Part print with two shaded views. Sizes in mm from the minimum x, y, z corner. Give positions to 0.01 mm unless a question says otherwise; leave off trailing zeros. Write each loop counter-clockwise with the first axis right and the second up, starting at its lowest first coordinate (ties: lowest second). Pieces come first, ordered by that corner, then holes.
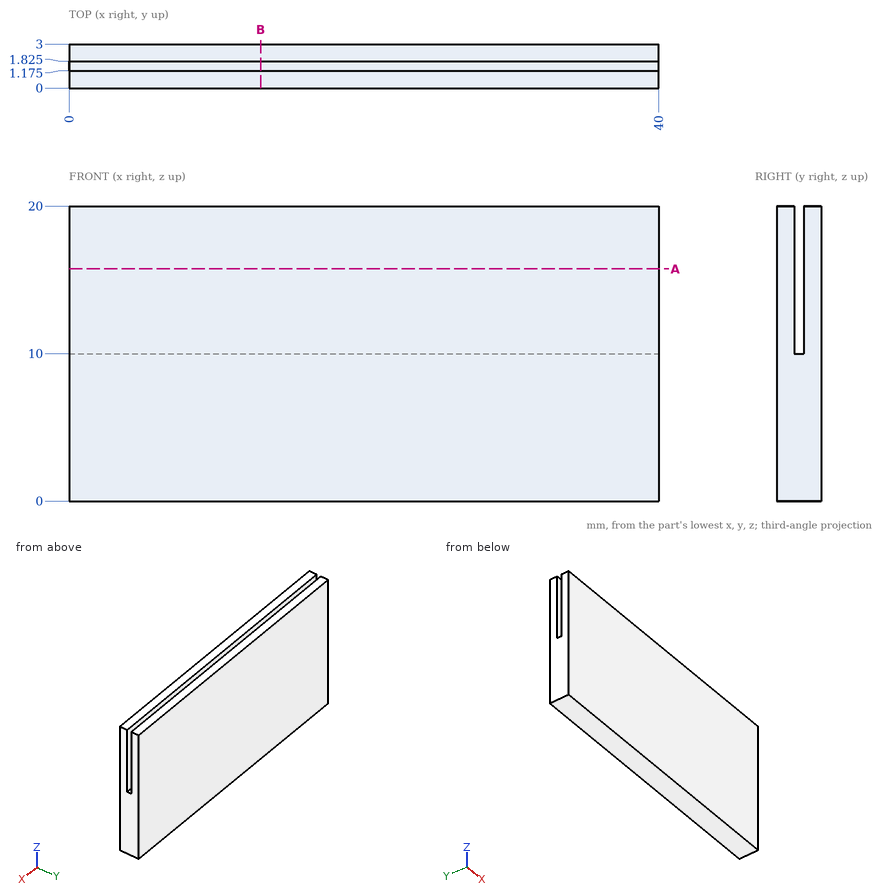
1) Saw through at B-B (x = 13). Write the cut outline in (y, z) (3 decimals), and give its area (3 significant figures).
Check result:
outline: (0, 0) - (3, 0) - (3, 20) - (1.825, 20) - (1.825, 10) - (1.175, 10) - (1.175, 20) - (0, 20) - close
area: 53.5 mm2
2) Saw through at A-A (z = 15.75). Write the cut outline in (x, y) (3 decimals), and give its area (3 significant figures).
Check result:
outline: (0, 0) - (40, 0) - (40, 1.175) - (0, 1.175) - close; (0, 1.825) - (40, 1.825) - (40, 3) - (0, 3) - close
area: 94.0 mm2
3) Flat gauge pins, fed straight in: P1, Ø1.5, axis at x = 30, y = 1, coming from the -Z side; P2, Ø0.5, axis at x = 16.5, y = 1.5, coming from the +Z side. Where does each tip first touch, or does it go through?
Check result:
P1: stops at z = 0
P2: stops at z = 10
4) Drill centre lines: L1, parallel to Y at x = 16.5, z = 10.25 (3 decimals); L2, parallel to Z at x = 24, y = 1.5. Where is each one in solid material? Low to high.
Check result:
L1: y = 0 to 1.175, 1.825 to 3
L2: z = 0 to 10
